from build123d import *

# Parameters (mm, degrees)
SKETCH1_R               = 4.7
BOSS_EXTRUDE1_DEPTH     = 11.866666667
SKETCH2_OUTSIDE_W       = 14.964
SKETCH2_OUTSIDE_H       = 14.964
SKETCH2_OUTSIDE_R       = 1.85
CUT_EXTRUDE1_DEPTH      = 3.5
BOSS_EXTRUDE2_START     = -8.366666667
BOSS_EXTRUDE2_DEPTH     = 8.366666667
FILLET1_R               = 0.5
FILLET2_R               = 0.5
SKETCH4_R               = 2.4
BOSS_EXTRUDE3_DEPTH     = 8.5
FILLET3_R               = 2
CHAMFER1_SIZE           = 0.5
CUT_EXTRUDE2_DEPTH      = 22.816361088
CUT_EXTRUDE2_DEPTH_BACK = 22.816361088
SKETCH5_R               = 1.275
BOSS_EXTRUDE4_START     = 3.5
BOSS_EXTRUDE4_DEPTH     = 8.366666667


# Read off the part's stored shape, not the designer's step: Boss-Extrude4
with BuildPart() as part:
    # Sketch1 → Boss-Extrude1 (new body)
    with BuildSketch(Plane.XY):
        Circle(SKETCH1_R)
    extrude(amount=BOSS_EXTRUDE1_DEPTH)

    # Sketch2 outside → Cut-Extrude1 (cut)
    with BuildSketch(Plane(origin=(0, 0, 0), x_dir=(-1, 0, 0), z_dir=(0, 0, -1))):
        Rectangle(SKETCH2_OUTSIDE_W, SKETCH2_OUTSIDE_H)
        Circle(SKETCH2_OUTSIDE_R, mode=Mode.SUBTRACT)
    extrude(amount=-CUT_EXTRUDE1_DEPTH, mode=Mode.SUBTRACT)

    # Sketch3 → Boss-Extrude2 (add)
    with BuildSketch(Plane.XY.offset(11.866666667).offset(BOSS_EXTRUDE2_START)):
        with BuildLine():
            Line((-1.5, 6.06733055), (-1.5, 4.45421149))
            ThreePointArc((-1.5, 4.45421149), (0, 4.7), (1.5, 4.45421149))
            Line((1.5, 4.45421149), (1.5, 6.06733055))
            ThreePointArc((1.5, 6.06733055), (0, 6.25), (-1.5, 6.06733055))
        make_face()
        with BuildLine():
            ThreePointArc((1.5, -4.45421149), (0, -4.7), (-1.5, -4.45421149))
            Line((-1.5, -4.45421149), (-1.5, -6.06733055))
            ThreePointArc((-1.5, -6.06733055), (0, -6.25), (1.5, -6.06733055))
            Line((1.5, -6.06733055), (1.5, -4.45421149))
        make_face()
    extrude(amount=BOSS_EXTRUDE2_DEPTH)

    # Fillet1
    fillet1_edges = [part.edges().sort_by_distance(p)[0] for p in [
        (-1.5, 6.06733055, 7.683333333),
        (-1.5, 4.45421149, 7.683333333),
        (1.5, 4.45421149, 7.683333333),
        (1.5, 6.06733055, 7.683333333),
        (1.5, -6.06733055, 7.683333333),
        (1.5, -4.45421149, 7.683333333),
        (-1.5, -4.45421149, 7.683333333),
        (-1.5, -6.06733055, 7.683333333),
    ]]
    fillet(fillet1_edges, radius=FILLET1_R)

    # Fillet2
    fillet2_edges = [part.edges().sort_by_distance(p)[0] for p in [
        (1.85, 0, 3.5),
    ]]
    fillet(fillet2_edges, radius=FILLET2_R)

    # Sketch4 → Boss-Extrude3 (add)
    with BuildSketch(Plane.XY.offset(11.866666667)):
        Circle(SKETCH4_R)
    extrude(amount=BOSS_EXTRUDE3_DEPTH)

    # Fillet3
    fillet3_edges = [part.edges().sort_by_distance(p)[0] for p in [
        (-2.4, 0, 11.866666667),
    ]]
    fillet(fillet3_edges, radius=FILLET3_R)

    # Chamfer1
    chamfer1_edges = [part.edges().sort_by_distance(p)[0] for p in [
        (-2.4, 0, 20.366666667),
        (1.85, 0, 0),
    ]]
    chamfer(chamfer1_edges, length=CHAMFER1_SIZE)

    # Sketch5 → Cut-Extrude2 (cut, two sides: drawn at the far end of the back side and taken through both)
    with BuildSketch(Plane(origin=(0, 0, 0), x_dir=(1, 0, 0), z_dir=(0, 1, 0)).offset(-CUT_EXTRUDE2_DEPTH_BACK)):
        with Locations(Location((0, -17.341666667, 0), (0, 0, 270))):
            Circle(SKETCH5_R)
    extrude(amount=CUT_EXTRUDE2_DEPTH + CUT_EXTRUDE2_DEPTH_BACK, mode=Mode.SUBTRACT)

    # Sketch6 → Cut-Revolve1 (revolve, cut)
    with BuildSketch(Plane(origin=(0, 0, 0), x_dir=(1, 0, 0), z_dir=(0, 1, 0)), mode=Mode.PRIVATE) as cut_revolve1_sk:
        Polygon((-4.7, -3.5), (-5.9, -3.5), (-5.9, -11.866666667), (-4.7, -11.866666667), (-3.4, -8.55965578), (-3.4, -3.5), align=None)
    revolve(cut_revolve1_sk.sketch.rotate(Axis((0, 0, 0), (0, 0, 1)), 180), axis=Axis((0, 0, 0), (0, 0, 1)), mode=Mode.SUBTRACT)


with BuildPart() as cut_revolve1_piece_1:
    # of the separate pieces the step leaves, piece 1, a body of its own (cut_revolve1_pieces)
    add(part.part.solids().sort_by_distance((2.4, 0, 19.866666667))[0])



with BuildPart() as cut_revolve1_piece_2:
    # of the separate pieces the step leaves, piece 2, a body of its own (cut_revolve1_pieces)
    add(part.part.solids().sort_by_distance((1.498035668, 5.706653059, 11.866666667))[0])


with BuildPart() as cut_revolve1_piece_3:
    # of the separate pieces the step leaves, piece 3, a body of its own (cut_revolve1_pieces)
    add(part.part.solids().sort_by_distance((1.498035668, -5.706653059, 11.866666667))[0])


with BuildPart() as cut_revolve1_piece_1_1:
    add(cut_revolve1_piece_1.part)

    add(cut_revolve1_piece_2.part)  # Boss-Extrude4 merges Cut-Revolve1 piece 2

    add(cut_revolve1_piece_3.part)  # Boss-Extrude4 merges Cut-Revolve1 piece 3
    # Boss-Extrude4 outline → Boss-Extrude4 (add)
    with BuildSketch(Plane.XY.offset(BOSS_EXTRUDE4_START)):
        with BuildLine():
            ThreePointArc((-1.498035668, -5.706653059), (0, -5.9), (1.498035668, -5.706653059))
            Line((1.498035668, -5.706653059), (1.498035668, -3.052194151))
            ThreePointArc((1.498035668, -3.052194151), (0, -3.4), (-1.498035668, -3.052194151))
            Line((-1.498035668, -3.052194151), (-1.498035668, -5.706653059))
        make_face()
        with BuildLine():
            Line((-1.498035668, 5.706653059), (-1.498035668, 3.052194151))
            ThreePointArc((-1.498035668, 3.052194151), (0, 3.4), (1.498035668, 3.052194151))
            Line((1.498035668, 3.052194151), (1.498035668, 5.706653059))
            ThreePointArc((1.498035668, 5.706653059), (0, 5.9), (-1.498035668, 5.706653059))
        make_face()
    extrude(amount=BOSS_EXTRUDE4_DEPTH)


solid = cut_revolve1_piece_1_1.part
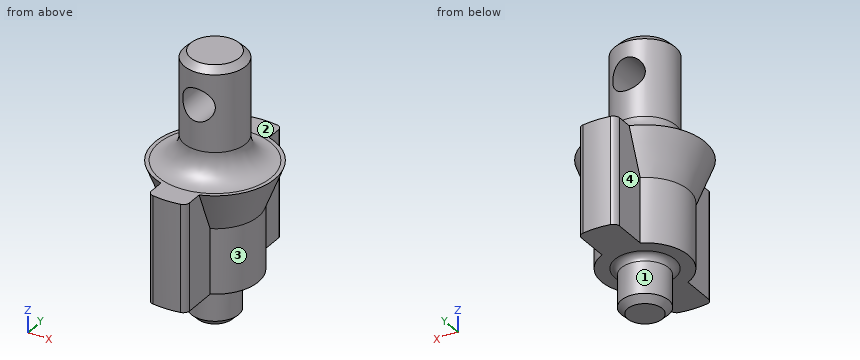
Design review of the part built by this model. Coordinates are the model's own, in mm. Face numbers are marked on the shaded views. A direction names the side the tool comes from. Coordinates: 2 decimals unless noted, no trailing zeros. Write each loop counter-clockwise with the first axis right and the second up, starting at its lowest first coordinate (ties: lowest second). Pieces come first, ordered by that corner, then holes. Notation, with made-up numbers: (6.25, 89) -> (17.25, 89) arc R16 cw to (17.25, 109) -> close; hole circle Ø1 at (-13, -17). An arc over 180 degrees is marked (long way). Write each question's results on one line, items separated by ' | '. Start each with the question number.
(1) Take a section at C-C on z = 6.25. Write out the cut boundary in (x, y).
(2) Take a section at A-A on x = 0. Write out the cut boundary in (y, z).
(3) For line 1 along Z through (x, y) = (0, 0.6); line 2 along X through (y, z) = (-0.5, 19.5); line 3 along X through (y, z) = (5.5, 5.5), list the stretches that pass through material, from the lowest coordinate up. Write a range as from..to.
(4) Tool access review of the marked faces 1, 2, 3 and 4: name each direction out of +Z, -Z, +X, -X, +Y, -Y from which nothing blocks a thin tool from reaching the whole face with its end or side.
(5) Take a section at D-D on y = -5. Write out the cut boundary in (x, z), and give its area (3 significant figures).
(6) Take a section at B-B on y = 0. Write out the cut boundary in (x, z) (3 decimals).
(7) Clearance check with flat-ended pins moving along their axes: P1, Ø0.8, axis at y = 4, z = 6.5, coming from the -X side; P2, Ø3, axis at y = -4, z = 8, coming from the +X side; P3, Ø4, axis at y = -3, z = 13.5, coming from the -X side; P4, Ø1, axis at x = 0.5, z = 17, coming from the +Y side. State where each tip first meets the part, or that it passes through.
Results found:
1) outline: (-1.5, -5.71) arc R0.5 ccw to (-1.09, -6.15) arc R6.25 ccw to (1.09, -6.15) arc R0.5 ccw to (1.5, -5.71) -> (1.5, -3.05) arc R3.4 ccw to (1.5, 3.05) -> (1.5, 5.71) arc R0.5 ccw to (1.09, 6.15) arc R6.25 ccw to (-1.09, 6.15) arc R0.5 ccw to (-1.5, 5.71) -> (-1.5, 3.05) arc R3.4 ccw to (-1.5, -3.05) -> close
2) outline: (-6.25, 3.5) -> (-2.35, 3.5) arc R0.5 cw to (-1.85, 3) -> (-1.85, 0.5) -> (-1.35, 0) -> (1.35, 0) -> (1.85, 0.5) -> (1.85, 3) arc R0.5 cw to (2.35, 3.5) -> (6.25, 3.5) -> (6.25, 11.87) -> (4.4, 11.87) arc R2 cw to (2.4, 13.87) -> (2.4, 16.07) -> (-2.4, 16.07) -> (-2.4, 13.87) arc R2 cw to (-4.4, 11.87) -> (-6.25, 11.87) -> close; (-2.4, 18.62) -> (2.4, 18.62) -> (2.4, 19.87) -> (1.9, 20.37) -> (-1.9, 20.37) -> (-2.4, 19.87) -> close
3) line 1: z = 0..16.07, 18.62..20.37 | line 2: x = -2.35..2.35 | line 3: x = -1.5..1.5
4) face 1: -Z | face 2: +Z | face 3: -Z, +X | face 4: -Z, -X, +Y
5) outline: (-1.5, 3.5) -> (1.5, 3.5) -> (1.5, 11.87) -> (-1.5, 11.87) -> close | area: 25.1 mm2
6) outline: (-4.7, 11.867) -> (-3.4, 8.56) -> (-3.4, 3.5) -> (-2.35, 3.5) arc R0.5 cw to (-1.85, 3) -> (-1.85, 0.5) -> (-1.35, 0) -> (1.35, 0) -> (1.85, 0.5) -> (1.85, 3) arc R0.5 cw to (2.35, 3.5) -> (3.4, 3.5) -> (3.4, 8.56) -> (4.7, 11.867) -> (4.4, 11.867) arc R2 cw to (2.4, 13.867) -> (2.4, 19.867) -> (1.9, 20.367) -> (-1.9, 20.367) -> (-2.4, 19.867) -> (-2.4, 13.867) arc R2 cw to (-4.4, 11.867) -> close; hole circle Ø2.55 at (0, 17.342)
7) P1: stops at x = -1.5 | P2: stops at x = 2.3 | P3: stops at x = -4.32 | P4: passes through
